```python
from build123d import *
from OCP.BRepFilletAPI import BRepFilletAPI_MakeChamfer

# Parameters (mm, degrees)
SKETCH1_W                      = 205
SKETCH1_H                      = 130
BOSS_EXTRUDE1_DEPTH            = 7.5
CHAMFER1_SIZE                  = 13
CHAMFER1_SIZE2                 = 7.505553499
SKETCH3_W                      = 68
SKETCH3_H                      = 67
BOSS_EXTRUDE2_DEPTH            = 62
CUT_EXTRUDE4_DEPTH             = 10
CUT_EXTRUDE4_DEPTH_BACK        = 63
SKETCH8_W                      = 57
SKETCH8_H                      = 57
SKETCH5_R                      = 11.5
SHAFT_1_DEPTH                  = 25
F_4_5_4_5_DIAMETER_HOLE1_D     = 4.5
F_4_5_4_5_DIAMETER_HOLE1_DEPTH = 5.829194732
SKETCH9_R                      = 11.5
SHAFT_2_DEPTH                  = 25
SUPPORT_START                  = 7.5
SUPPORT_STRUCTURE_DEPTH        = 62
F_4_5_4_5_DIAMETER_HOLE2_D     = 4.5
F_4_5_4_5_DIAMETER_HOLE2_DEPTH = 5.829194732
SKETCH15_R                     = 11.5
SHAFT_3_DEPTH                  = 25
F_4_5_4_5_DIAMETER_HOLE3_D     = 4.5
F_4_5_4_5_DIAMETER_HOLE3_DEPTH = 5.829194732
CUT_EXTRUDE3_REACH             = 169.449
SKETCH18_R                     = 19.1
F_4_5_4_5_DIAMETER_HOLE4_D     = 4.5
CIRPATTERN1_START              = -42
CIRPATTERN1_OUTLINE_R          = 2.25
CIRPATTERN1_DEPTH              = 5
LPATTERN1_COUNT                = 2
LPATTERN1_PITCH                = 12


# Read off the part's stored shape, not the designer's step: Support Structure, CirPattern1
with BuildPart() as part:
    # Sketch1 → Boss-Extrude1 (new, symmetric)
    with BuildSketch(Plane(origin=(0, 0, 0), x_dir=(1, 0, 0), z_dir=(0, 1, 0))):
        with Locations((-17.5, 0)):
            Rectangle(SKETCH1_W, SKETCH1_H)
    extrude(amount=BOSS_EXTRUDE1_DEPTH, both=True)

    # Chamfer1: one chamfer whose edges measure the first distance from different faces: ONE call of the kernel's chamfer builder (chamfer() names one face for all edges)
    chamfer1_edges_1 = [part.edges().sort_by_distance(p)[0] for p in [
        (-120, 7.5, 0),
    ]]
    chamfer1_side_1 = [part.faces().sort_by_distance(p)[0] for p in [
        (-120, 0, 0),
    ]]
    chamfer1_edges_2 = [part.edges().sort_by_distance(p)[0] for p in [
        (-17.5, 7.5, 65),
    ]]
    chamfer1_side_2 = [part.faces().sort_by_distance(p)[0] for p in [
        (-17.5, 0, 65),
    ]]
    chamfer1_edges_3 = [part.edges().sort_by_distance(p)[0] for p in [
        (85, 7.5, 0),
    ]]
    chamfer1_side_3 = [part.faces().sort_by_distance(p)[0] for p in [
        (85, 0, 0),
    ]]
    chamfer1_edges_4 = [part.edges().sort_by_distance(p)[0] for p in [
        (-17.5, 7.5, -65),
    ]]
    chamfer1_side_4 = [part.faces().sort_by_distance(p)[0] for p in [
        (-17.5, 0, -65),
    ]]
    chamfer1 = BRepFilletAPI_MakeChamfer(part.part.solid().wrapped)
    for e in chamfer1_edges_1:
        chamfer1.Add(CHAMFER1_SIZE, CHAMFER1_SIZE2, e.wrapped, chamfer1_side_1[0].wrapped)  # the first distance lies on this face
    for e in chamfer1_edges_2:
        chamfer1.Add(CHAMFER1_SIZE, CHAMFER1_SIZE2, e.wrapped, chamfer1_side_2[0].wrapped)  # the first distance lies on this face
    for e in chamfer1_edges_3:
        chamfer1.Add(CHAMFER1_SIZE, CHAMFER1_SIZE2, e.wrapped, chamfer1_side_3[0].wrapped)  # the first distance lies on this face
    for e in chamfer1_edges_4:
        chamfer1.Add(CHAMFER1_SIZE, CHAMFER1_SIZE2, e.wrapped, chamfer1_side_4[0].wrapped)  # the first distance lies on this face
    add(Compound.cast(chamfer1.Shape()), mode=Mode.REPLACE)

    # Sketch3 → Boss-Extrude2 (add)
    with BuildSketch(Plane(origin=(0, 7.5, 0), x_dir=(1, 0, 0), z_dir=(0, 1, 0))):
        with Locations((-71, 7.5)):
            Rectangle(SKETCH3_W, SKETCH3_H)
    extrude(amount=BOSS_EXTRUDE2_DEPTH)

    # Sketch8 → Cut-Extrude4 (cut, two sides: drawn at the far end of the back side and taken through both)
    with BuildSketch(Plane.ZY.offset(105).offset(-CUT_EXTRUDE4_DEPTH_BACK)):
        with Locations((-7.5, 36)):
            Rectangle(SKETCH8_W, SKETCH8_H)
    extrude(amount=CUT_EXTRUDE4_DEPTH + CUT_EXTRUDE4_DEPTH_BACK, mode=Mode.SUBTRACT)

    # Sketch5 → Shaft 1 (add)
    with BuildSketch(Plane(origin=(0, 7.5, 0), x_dir=(1, 0, 0), z_dir=(0, 1, 0))):
        with Locations(Location((60, 32.5, 0), (0, 0, 90))):
            Circle(SKETCH5_R)
        with BuildLine():
            Line((56.825, 38.171805268), (63.175, 38.171805268))
            ThreePointArc((63.175, 38.171805268), (60, 26), (56.825, 38.171805268))
        make_face(mode=Mode.SUBTRACT)
    extrude(amount=SHAFT_1_DEPTH)

    # Ø4.5 (4.5) Diameter Hole1
    with Locations(Plane.XY.offset(-38.171805268)):
        with Locations((60, 26)):
            f_4_5_4_5_diameter_hole1 = Hole(F_4_5_4_5_DIAMETER_HOLE1_D / 2, depth=F_4_5_4_5_DIAMETER_HOLE1_DEPTH)

    # Sketch9 → Shaft 2 (add)
    with BuildSketch(Plane(origin=(0, 69.5, 0), x_dir=(1, 0, 0), z_dir=(0, 1, 0))):
        with Locations(Location((-60, 32.5, 0), (0, 0, 47.657394548))):
            Circle(SKETCH9_R)
        with BuildLine():
            Line((-63.175, 38.171805268), (-56.825, 38.171805268))
            ThreePointArc((-56.825, 38.171805268), (-60, 26), (-63.175, 38.171805268))
        make_face(mode=Mode.SUBTRACT)
    extrude(amount=SHAFT_2_DEPTH)

    # Support Structure outline → Support Structure (add)
    with BuildSketch(Plane(origin=(0, 0, 0), x_dir=(1, 0, 0), z_dir=(0, 1, 0)).offset(SUPPORT_START)):
        with BuildLine():
            Line((-67.745966692, 41), (-52.254033308, 41))
            ThreePointArc((-52.254033308, 41), (-60, 44), (-67.745966692, 41))
        make_face()
    extrude(amount=SUPPORT_STRUCTURE_DEPTH)

    # Ø4.5 (4.5) Diameter Hole2
    with Locations(Plane.XY.offset(-38.171805268)):
        with Locations((-60, 88)):
            f_4_5_4_5_diameter_hole2 = Hole(F_4_5_4_5_DIAMETER_HOLE2_D / 2, depth=F_4_5_4_5_DIAMETER_HOLE2_DEPTH)

    # Sketch15 → Shaft 3 (add)
    with BuildSketch(Plane(origin=(0, 7.5, 0), x_dir=(1, 0, 0), z_dir=(0, 1, 0))):
        with Locations(Location((0, -37.5, 0), (0, 0, 90))):
            Circle(SKETCH15_R)
        with BuildLine():
            Line((3.175, -43.171805268), (-3.175, -43.171805268))
            ThreePointArc((-3.175, -43.171805268), (0, -31), (3.175, -43.171805268))
        make_face(mode=Mode.SUBTRACT)
    extrude(amount=SHAFT_3_DEPTH)

    # Ø4.5 (4.5) Diameter Hole3
    with Locations(Plane(origin=(0, 0, 43.171805268), x_dir=(-1, 0, 0), z_dir=(0, 0, -1))):
        with Locations((0, 26)):
            f_4_5_4_5_diameter_hole3 = Hole(F_4_5_4_5_DIAMETER_HOLE3_D / 2, depth=F_4_5_4_5_DIAMETER_HOLE3_DEPTH)

    # Sketch18 → Cut-Extrude3 (cut, up to next)
    with BuildSketch(Plane(origin=(-37, 0, 0), x_dir=(0, 0, -1), z_dir=(1, 0, 0)), mode=Mode.PRIVATE) as cut_extrude3_sk1:
        with Locations((7.5, 38.5)):
            Circle(SKETCH18_R)
    cut_extrude3_tool1 = extrude(cut_extrude3_sk1.sketch, amount=-CUT_EXTRUDE3_REACH, mode=Mode.PRIVATE) & part.part
    add(cut_extrude3_tool1.solids().sort_by_distance((-37, 38.5, -7.5))[0], mode=Mode.SUBTRACT)

    # Ø4.5 (4.5) Diameter Hole4 (through all)
    with Locations(Plane(origin=(-37, 0, 0), x_dir=(0, 0, -1), z_dir=(1, 0, 0))):
        with Locations((31.05, 62.05)):
            Hole(F_4_5_4_5_DIAMETER_HOLE4_D / 2)

    # CirPattern1 outline → CirPattern1 (cut)
    with BuildSketch(Plane.YZ.offset(CIRPATTERN1_START)):
        with Locations((62.05, 16.05)):
            Circle(CIRPATTERN1_OUTLINE_R)
        with Locations((14.95, 16.05)):
            Circle(CIRPATTERN1_OUTLINE_R)
        with Locations((14.95, -31.05)):
            Circle(CIRPATTERN1_OUTLINE_R)
    extrude(amount=CIRPATTERN1_DEPTH, mode=Mode.SUBTRACT)

    # LPattern1: Ø4.5 (4.5) Diameter Hole1, Ø4.5 (4.5) Diameter Hole2, Ø4.5 (4.5) Diameter Hole3 ×2
    with Locations(*[(0, -i * LPATTERN1_PITCH, 0) for i in range(1, LPATTERN1_COUNT)]):
        add(f_4_5_4_5_diameter_hole1, mode=Mode.SUBTRACT)
        add(f_4_5_4_5_diameter_hole2, mode=Mode.SUBTRACT)
        add(f_4_5_4_5_diameter_hole3, mode=Mode.SUBTRACT)


solid = part.part
```
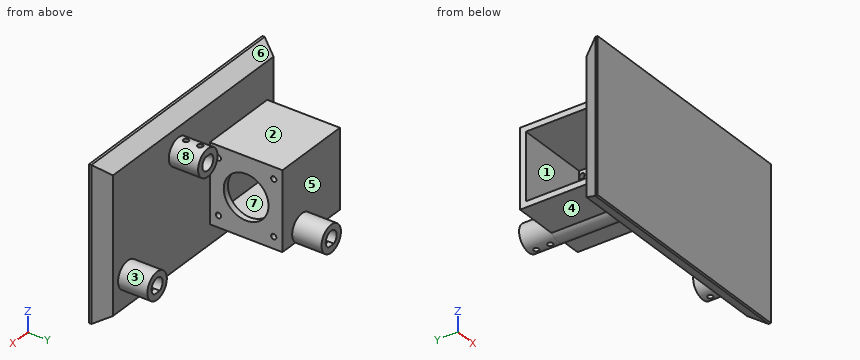
Can you work these out from the model? Positions are in its coordinate system, mm. Face numbers are marked on the shaded views. A direction names the side the tool comes from. Give positions to 0.01 mm unless a question says otherwise; leave off trailing zeros. Write each loop counter-clockwise with the first axis right and the second up, starting at its lowest first coordinate (ties: lowest second). Pieces come first, ordered by that corner, then holes. Notation, with made-up numbers: (22, 24) -> (70, 24) arc R27 cw to (70, 53) -> close; hole circle Ø4 at (-12, 89.25). An arc over 180 degrees is marked (long way). Write item = value, one per line.
(1) Suppose I cut it at D-D on z = -18. Write out the boundary of the cut face in (x, y), then the cut area to 3 significant figures.
Worked out:
outline = (-120, -7.5) -> (85, -7.5) -> (85, -5.5) -> (77.49, 7.5) -> (-37, 7.5) -> (-37, 22.55) -> (-42, 22.55) -> (-42, 7.5) -> (-112.49, 7.5) -> (-120, -5.5) -> close; (-105, 64.5) -> (-42, 64.5) -> (-42, 54.45) -> (-37, 54.45) -> (-37, 69.5) -> (-105, 69.5) -> close
area = 3,440 mm^2
(2) Suppose I cut it at C-C on x = 0. Write out the boundary of the cut face in (y, z), then the cut area to 3 significant figures.
Worked out:
outline = (-7.5, -65) -> (-5.5, -65) -> (7.5, -57.49) -> (7.5, 26) -> (32.5, 26) -> (32.5, 31) -> (7.5, 31) -> (7.5, 43.17) -> (11.75, 43.17) -> (11.75, 49) -> (7.5, 49) -> (7.5, 57.49) -> (-5.5, 65) -> (-7.5, 65) -> close; (16.25, 43.17) -> (23.75, 43.17) -> (23.75, 49) -> (16.25, 49) -> close; (28.25, 43.17) -> (32.5, 43.17) -> (32.5, 49) -> (28.25, 49) -> close
area = 2,070 mm^2
(3) Suppose I cut it at B-B on y = 62.05. Write out the boundary of the cut face in (x, z), then the cut area to 3 significant figures.
Worked out:
outline = (-105, -41) -> (-67.75, -41) arc R11.5 ccw to (-52.25, -41) -> (-37, -41) -> (-37, -33.3) -> (-42, -33.3) -> (-42, -36) -> (-105, -36) -> close; (-105, 21) -> (-42, 21) -> (-42, 18.3) -> (-37, 18.3) -> (-37, 26) -> (-105, 26) -> close; (-42, -28.8) -> (-37, -28.8) -> (-37, 13.8) -> (-42, 13.8) -> close
area = 952 mm^2
(4) I'm going to push flat-ended pins straight in: P1, Ø5, axis at x = -90, y = 11, coming from the -Z side; P2, Ø3.5, axis at x = -60, y = 88, coming from the -Z side; P3, Ø10, axis at y = 14.5, z = 27.5, coming from the +X side; P4, Ø2.5, axis at y = 62.05, z = 16.05, coming from the +X side. Where does each tip first touch, or does it pass through?
Worked out:
P1 = -41
P2 = -26.24
P3 = 10.36
P4 = through
(5) Suppose I cut it at A-A on x = -60. Write out the boundary of the cut face in (y, z), then the cut area to 3 significant figures.
Worked out:
outline = (-7.5, -65) -> (-5.5, -65) -> (7.5, -57.49) -> (7.5, -44) -> (73.75, -44) -> (73.75, -38.17) -> (69.5, -38.17) -> (69.5, -26) -> (94.5, -26) -> (94.5, -21) -> (69.5, -21) -> (69.5, 26) -> (7.5, 26) -> (7.5, 57.49) -> (-5.5, 65) -> (-7.5, 65) -> close; (78.25, -44) -> (85.75, -44) -> (85.75, -38.17) -> (78.25, -38.17) -> close; (90.25, -44) -> (94.5, -44) -> (94.5, -38.17) -> (90.25, -38.17) -> close; hole (7.5, -36) -> (64.5, -36) -> (64.5, 21) -> (7.5, 21) -> close
area = 3,160 mm^2
(6) I need wall thicknesses on probe 1 along Y at (x, z) = (-39.8, -7.5); probe 2 along X at (y, z) = (83.5, -32.5); probe 3 along Z at (x, y) = (-68, 13). Which ranges of each line are inside material? Lowest first, please. Write a range as from..to.
Worked out:
probe_1 = -7.5..19.4, 57.6..69.5
probe_2 = -71.5..-66.5, -53.5..-48.5
probe_3 = -41..-36, 21..26
(7) Thinking about a two-plate mould opening in Z: for the marked faces 5, 6, 7 and 8, which applies, released by +Z, released by -Z, zero draft, split by the parting line, or undercut?
Worked out:
face_5 = zero draft
face_6 = released by +Z
face_7 = undercut
face_8 = split by the parting line
(8) For the marked faces 1, 2, 3 and 4, which set-ups out of +Z, -Z, +X, -X, +Y, -Y let a thin tool reach every point of the face, with its end or its side?
Worked out:
face_1 = -X
face_2 = +Z, -X, +Y
face_3 = +Y
face_4 = -Z, -X, +Y
